Could you check a few things on this drawing? It's one solid part, dimensions in mm from its lowest x, y, z. A direction names the side the tool comes from. Give positions to 0.01 mm unless a question says otherwise; leave off trailing zeros. Order: outer loops, then holes, each group sorted by start corner. A loop starts at its lowest first (then second) coordinate and runs counter-clockwise, first axis right, second up. Notation, with made-up numbers: (9.25, 80) -> (43.25, 80) arc R20 ccw to (43.25, 93) -> close; hole circle Ø8 at (31.25, 23). An arc over 180 degrees is marked (long way). Write each question's results on one line, items separated by ' | '. Start each with the question number.
Q1. Imagine slicing it at A-A, the plane x = 59. Please give me the cut outline in (y, z).
Q2. I'm going to push a flat-ended pin straight in: pin 1 (16 mm diameter, centred on x = 87.5, z = 71.5, fed in from -Y). Where does the tip first touch, or does it pass through?
Q3. Imagine slicing it at B-B, the plane y = 30.5. Please give me the cut outline in (x, z).
Q4. I need wall thicknesses on line 1 along Z through (x, y) = (41, 15); line 2 along X through (y, z) = (26.5, 26); line 3 along Y through (x, z) = (83, 69). Which ranges of each line are inside material? Lowest first, please. Write a range as [from, to].
Q5. For the marked faces 1, 2 and 3, which set-ups out of +Z, -Z, +X, -X, +Y, -Y let a thin tool reach every point of the face, with its end or its side?
Q6. Thinking about a two-plate mould opening in Z: for the marked faces 4, 5 and 6, which applies, pulls with the +Z half, pulls with the -Z half, needs draft (parallel to the pull), parting line crosses it, or undercut?
Q7. Imagine slicing it at D-D, the plane x = 40. Please give me the cut outline in (y, z).
Q8. Imagine slicing it at C-C, the plane z = 57.5. Please give me the cut outline in (x, y), then the cut area to 3 significant figures.
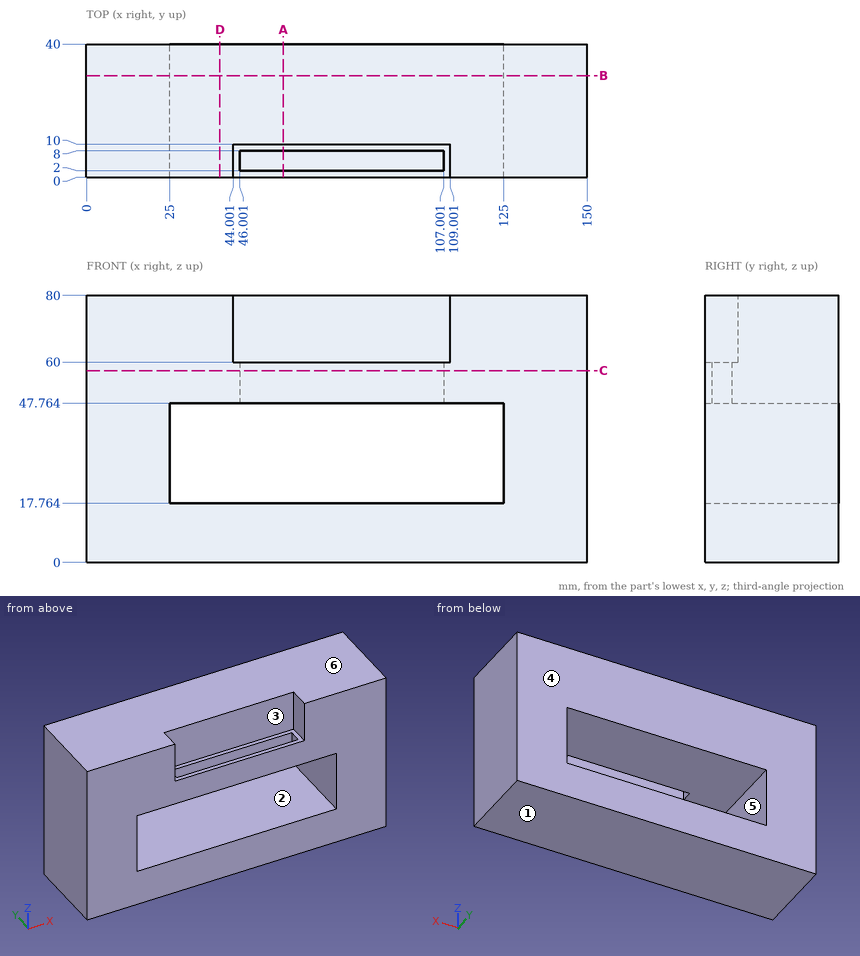
Geometry check:
1) outline: (0, 0) -> (40, 0) -> (40, 17.76) -> (0, 17.76) -> close; (0, 47.76) -> (2, 47.76) -> (2, 60) -> (0, 60) -> close; (8, 47.76) -> (40, 47.76) -> (40, 80) -> (10, 80) -> (10, 60) -> (8, 60) -> close
2) pin 1: y = 10
3) outline: (0, 0) -> (150, 0) -> (150, 80) -> (0, 80) -> close; hole (25, 17.76) -> (125, 17.76) -> (125, 47.76) -> (25, 47.76) -> close
4) line 1: [0, 17.76], [47.76, 80] | line 2: [0, 25], [125, 150] | line 3: [10, 40]
5) face 1: -Z, +X, -X, +Y, -Y | face 2: +Y, -Y | face 3: +Z, -Y
6) face 4: needs draft | face 5: undercut | face 6: pulls with the +Z half
7) outline: (0, 0) -> (40, 0) -> (40, 17.76) -> (0, 17.76) -> close; (0, 47.76) -> (40, 47.76) -> (40, 80) -> (0, 80) -> close
8) outline: (0, 0) -> (150, 0) -> (150, 40) -> (0, 40) -> close; hole (46, 2) -> (107, 2) -> (107, 8) -> (46, 8) -> close | area: 5,630 mm²
